from build123d import *

# Parameters (mm, degrees)
BOSS_EXTRUDE1_DEPTH         = 125
SKETCH1_3_R                 = 12.5
BOSS_EXTRUDE2_DEPTH         = 65
SKETCH1_4_R                 = 60
SKETCH1_4_R_2               = 8
SKETCH1_4_R_3               = 30
BOSS_EXTRUDE3_DEPTH         = 35
BOSS_EXTRUDE4_START         = -46
BOSS_EXTRUDE4_DEPTH         = 32
FILLET1_RADIUS              = 16
FILLET1_LENGTH              = 30
F_16_0MM_DOWEL_HOLE1_D      = 16
FILLET1_OF_MIRROR1_2_RADIUS = 16
FILLET1_OF_MIRROR1_2_LENGTH = 30
SKETCH4_R                   = 55
CUT_EXTRUDE1_DEPTH          = 15


with BuildPart() as part:
    # Sketch1 → Boss-Extrude1 (new body)
    with BuildSketch(Plane.XY):
        with BuildLine():
            ThreePointArc((20, 0), (0, -20), (-20, 0))
            Line((-20, 0), (-30, 0))
            ThreePointArc((-30, 0), (0, -30), (30, 0))
            Line((30, 0), (20, 0))
        make_face()
    extrude(amount=BOSS_EXTRUDE1_DEPTH)

    # Sketch1<3> → Boss-Extrude2 (add)
    with BuildSketch(Plane.XY):
        with BuildLine():
            Line((-30, 0), (-20, 0))
            ThreePointArc((-20, 0), (0, -20), (20, 0))
            Line((20, 0), (30, 0))
            ThreePointArc((30, 0), (0, 30), (-30, 0))
        make_face()
        Circle(SKETCH1_3_R, mode=Mode.SUBTRACT)
    extrude(amount=BOSS_EXTRUDE2_DEPTH)

    # Sketch1<4> → Boss-Extrude3 (add)
    with BuildSketch(Plane.XY):
        Circle(SKETCH1_4_R)
        with Locations((0, 42)):
            Circle(SKETCH1_4_R_2, mode=Mode.SUBTRACT)
        with Locations((-42, 0)):
            Circle(SKETCH1_4_R_2, mode=Mode.SUBTRACT)
        with Locations((0, -42)):
            Circle(SKETCH1_4_R_2, mode=Mode.SUBTRACT)
        with Locations((42, 0)):
            Circle(SKETCH1_4_R_2, mode=Mode.SUBTRACT)
        Circle(SKETCH1_4_R_3, mode=Mode.SUBTRACT)
    extrude(amount=BOSS_EXTRUDE3_DEPTH)

    # Sketch2 → Boss-Extrude4 (add)
    with BuildSketch(Plane.XY.offset(125).offset(BOSS_EXTRUDE4_START)):
        with BuildLine():
            Line((60, 0), (30, 0))
            ThreePointArc((30, 0), (21.213203436, -21.213203436), (0, -30))
            Line((0, -30), (60, -30))
            Line((60, -30), (60, 0))
        make_face()
    boss_extrude4 = extrude(amount=BOSS_EXTRUDE4_DEPTH)

    # Fillet1: full round fillet: the end face becomes a half cylinder, R = half its width
    fillet1_face = Plane((60, -15, 95), x_dir=(0, -1, 0), z_dir=(1, 0, 0))  # on the end face: x along it, z out of the body
    fillet1_slab = fillet1_face.offset(-FILLET1_RADIUS / 2) * Box(FILLET1_LENGTH, 2 * FILLET1_RADIUS, FILLET1_RADIUS, mode=Mode.PRIVATE)  # the body's end, R deep
    fillet1_round = Plane((44, -15, 95), x_dir=(1, 0, 0), z_dir=(0, -1, 0)) * Cylinder(FILLET1_RADIUS, FILLET1_LENGTH, mode=Mode.PRIVATE)  # its axis R under the face
    add(fillet1_slab - fillet1_round, mode=Mode.SUBTRACT)

    # Ø16.0mm Dowel Hole1 (through all)
    with Locations(Plane(origin=(44, 0, 95), x_dir=(0, 0, 1), z_dir=(0, 1, 0))):
        with Locations((0, 0)):
            f_16_0mm_dowel_hole1 = Hole(F_16_0MM_DOWEL_HOLE1_D / 2)

    # Mirror1: Boss-Extrude4, Ø16.0mm Dowel Hole1 across plane
    add(boss_extrude4.mirror(Plane(origin=(0, 0, 0), x_dir=(0, 0, 1), z_dir=(1, 0, 0))))
    add(f_16_0mm_dowel_hole1.mirror(Plane(origin=(0, 0, 0), x_dir=(0, 0, 1), z_dir=(1, 0, 0))), mode=Mode.SUBTRACT)

    # Fillet1 of Mirror1 2: full round fillet: the end face becomes a half cylinder, R = half its width
    fillet1_of_mirror1_2_face = Plane((-60, -15, 95), x_dir=(0, -1, 0), z_dir=(-1, 0, 0))  # on the end face: x along it, z out of the body
    fillet1_of_mirror1_2_slab = fillet1_of_mirror1_2_face.offset(-FILLET1_OF_MIRROR1_2_RADIUS / 2) * Box(FILLET1_OF_MIRROR1_2_LENGTH, 2 * FILLET1_OF_MIRROR1_2_RADIUS, FILLET1_OF_MIRROR1_2_RADIUS, mode=Mode.PRIVATE)  # the body's end, R deep
    fillet1_of_mirror1_2_round = Plane((-44, -15, 95), x_dir=(-1, 0, 0), z_dir=(0, -1, 0)) * Cylinder(FILLET1_OF_MIRROR1_2_RADIUS, FILLET1_OF_MIRROR1_2_LENGTH, mode=Mode.PRIVATE)  # its axis R under the face
    add(fillet1_of_mirror1_2_slab - fillet1_of_mirror1_2_round, mode=Mode.SUBTRACT)

    # Sketch4 → Cut-Extrude1 (cut)
    with BuildSketch(Plane(origin=(0, 0, 0), x_dir=(-1, 0, 0), z_dir=(0, 0, -1))):
        Circle(SKETCH4_R)
    extrude(amount=-CUT_EXTRUDE1_DEPTH, mode=Mode.SUBTRACT)


solid = part.part
Can you work these out from the model? Positions are in its coordinate system, mm. A direction names the side the tool comes from. Round coordinates to 2 decimals unless told otherwise and drop trailing zeros. Write each loop counter-clockwise with the first axis right and the second up, starting at its lowest first coordinate (ties: lowest second). Pieces come first, ordered by that corner, then holes. Notation, with made-up numbers: M 82.25,47 L 102.25,47 A19 ccw 102.25,67 Z; hole C 54.5,86.5 d10. An arc over 180 degrees is marked long. Use CSV: the item, a comma, the result in double quotes.
(1) Imagine slicing it at B-B (y = 47). Write out the boundary of the cut face in (x, z) (3 decimals).
Check values:
outline,"M -37.296,0 L -28.566,0 L -28.566,15 L -6.245,15 L -6.245,35 L -37.296,35 Z; M 6.245,15 L 28.566,15 L 28.566,0 L 37.296,0 L 37.296,35 L 6.245,35 Z"
(2) We'd pull the mould along Y, two halves only. Please class faces 1 (the cylindrical face through (11.923, -53.692, 7.395)), 2 (the cylindrical face through (0, -20, 95)), 3 (the flat face through (31, -18, 111)): +Y half, -Y half, draft (parallel to the pull), parting line (faces both ways), or undercut.
Check values:
face 1,"undercut"
face 2,"+Y half"
face 3,"draft"
(3) On a 3-axis mill with a long thin cutter (end or side, diameter ignored), from which of +Z, -Z, +X, -X, +Y, -Y can I reach the whole of each face in a straight line? I mean faces 4 (the flat face through (-31, -18, 111)), 5 (the flat face through (-7, 11, 65)), 6 (the flat face through (31, -18, 79)), 7 (the cylindrical face through (-48.349, -4.868, 24.86)), 8 (the flat face through (1, -30, 95)). Say none if no direction works.
Check values:
face 4,"+Z, -X, -Y"
face 5,"+Z, +Y"
face 6,"+X, -Y"
face 7,"-Z"
face 8,"+Z, +X, -X, -Y"
(4) I'm going to push flat-ended pins straight in: pin 1 (9 mm diameter, centred on x = -21.5, y = -10, fed in from -Z); pin 2 (20 mm diameter, centred on x = -36.5, z = 81, fed in from +Y); pin 3 (1 mm diameter, centred on x = 39.5, z = 13, fed in from +Y). Where does each tip first touch, or does it pass through?
Check values:
pin 1,"z = 15"
pin 2,"y = 0"
pin 3,"y = 45.6"
(5) Imagine slicing it at C-C (x = -42). Write out the boundary of the cut face in (y, z), plus the area to 3 significant figures.
Check values:
outline,"M -42.85,0 L -35.51,0 L -35.51,15 L -8,15 L -8,35 L -42.85,35 Z; M -30,79 L 0,79 L 0,87.25 L -30,87.25 Z; M -30,102.75 L 0,102.75 L 0,111 L -30,111 Z; M 8,15 L 35.51,15 L 35.51,0 L 42.85,0 L 42.85,35 L 8,35 Z"
area,"2,110 mm^2"
(6) Imagine slicing it at A-A (z = 95). Write out the boundary of the cut face in (x, y).
Check values:
outline,"M -60,-30 L -52,-30 L -52,0 L -60,0 Z; M -36,-30 L 36,-30 L 36,0 L 20,0 A20 cw -20,0 L -36,0 Z; M 52,-30 L 60,-30 L 60,0 L 52,0 Z"
(7) Imagine slicing it at D-D (y = -16). Write out the boundary of the cut face in (x, z), plus the area to 3 significant figures.
Check values:
outline,"M -57.83,0 L -52.62,0 L -52.62,15 L 52.62,15 L 52.62,0 L 57.83,0 L 57.83,35 L 25.38,35 L 25.38,79 L 44,79 A16 ccw 44,111 L 25.38,111 L 25.38,125 L 12,125 L 12,65 L -12,65 L -12,125 L -25.38,125 L -25.38,111 L -44,111 A16 ccw -44,79 L -25.38,79 L -25.38,35 L -57.83,35 Z; hole C -44,95 d16; hole C 44,95 d16"
area,"7,190 mm^2"
(8) I need wall thicknesses on line 1 along Y through (x, z) = (0, 20.5); line 2 along Z through (x, y) = (-22, -22.5); line 3 along Y through (x, z) = (0, 43.5). Which ranges of each line are inside material? Lowest first, please.
Check values:
line 1,"-60 to -50, -34 to -12.5, 12.5 to 34, 50 to 60"
line 2,"15 to 35, 79 to 111"
line 3,"-30 to -12.5, 12.5 to 30"
